Model file for the job. Use its own axes, mm. A direction names the side the tool comes from. Coordinates: 2 decimals unless noted, no trailing zeros. Write each loop counter-clockwise with the first axis right and the second up, starting at its lowest first coordinate (ties: lowest second). Pieces come first, ordered by that corner, then holes. Notation, with made-up numbers: (68, -39) - (109, -39) arc R14 ccw to (109, -12) - close; hole circle Ø11 at (-13.75, -9). An arc over 180 degrees is marked (long way). Put each result on its own line as item: value. Start each with the question number.
1. Which spindle directions (+Z, -Z, +X, -X, +Y, -Y) get a long thin tool onto all of the face, cutting with end or side? Do faces 4 (the face through (-3.53, 4.97, -17.61)), 5 (the face through (2, -2, -13)), 6 (the face through (-2.24, 4.97, -16.63)). Say none if no direction does.
2. Saw through at D-D, the plane x = -1.5. Write the cut outline in (y, z), plus the area to 3 significant figures.
3. Saw through at A-A, the plane x = 0. Write the cut outline in (y, z), plus the area to 3 significant figures.
4. Saw through at B-B, the plane y = 0. Write the cut outline in (x, z).
5. Drill centre lines: L1, parallel to Y at x = 3.5, z = -17; L2, parallel to Z at x = 0, y = -3.9; L3, parallel to Y at x = 2.75, z = -13. Where is each one in solid material? Low to high. Write a range as from..to.
6. Drop flat-ended pins along their axis: P1, Ø1.5, axis at x = -1.5, y = -3, coming from the -Z side; P2, Ø1.5, axis at y = 5, z = -3, coming from the +X side; P3, Ø1.5, axis at x = 1.5, y = -1.5, coming from the -Z side. Give the stop position or say it passes through.
7. Saw through at C-C, the plane z = 4. Write the cut outline in (x, y).
8. Pull direction Y, two halves, no side cores. Call faces 1 (the face through (5.6, 5, -5.1)), 2 (the face through (-0.759, -2.507, -11.583)), 3 (the face through (5.1, -3.2, -16.4)): released by +Y, released by -Y, zero draft, split by the parting line, or undercut.
```python
from build123d import *

# Parameters (mm, degrees)
SKETCH1_W               = 14
SKETCH1_H               = 15
BOSS_EXTRUDE1_DEPTH     = 7
SKETCH3_R               = 4
CUT_EXTRUDE1_DEPTH      = 16
SKETCH4_W               = 14
SKETCH4_H               = 14
BOSS_EXTRUDE2_DEPTH     = 12
SKETCH7_R               = 6
CUT_EXTRUDE7_DEPTH      = 3
SKETCH8_R               = 2.5
CUT_EXTRUDE8_DEPTH      = 11
CUT_EXTRUDE8_DEPTH_BACK = 5
SKETCH9_W               = 4.5
SKETCH9_H               = 6
CUT_EXTRUDE9_DEPTH      = 8
CUT_EXTRUDE9_DEPTH_BACK = 8
CHAMFER1_SIZE           = 5
SKETCH13_R              = 3.5
SKETCH13_R_2            = 2.5
BOSS_EXTRUDE3_DEPTH     = 1
CUT_EXTRUDE10_DEPTH     = 6
CHAMFER2_SIZE           = 4
CHAMFER2_SIZE2          = 2.800830153
CHAMFER2_PART_2_SIZE    = 4
CHAMFER2_PART_2_SIZE2   = 2.800830153
CHAMFER3_SIZE           = 4
CHAMFER3_SIZE2          = 2.800830153
CHAMFER3_PART_2_SIZE    = 4
CHAMFER3_PART_2_SIZE2   = 2.800830153
FILLET1_R               = 1
FILLET2_R               = 4


with BuildPart() as part:
    # Sketch1 → Boss-Extrude1 (new body, symmetric)
    with BuildSketch(Plane(origin=(0, 0, 0), x_dir=(1, 0, 0), z_dir=(0, 1, 0))):
        Rectangle(SKETCH1_W, SKETCH1_H)
    extrude(amount=BOSS_EXTRUDE1_DEPTH, both=True)

    # Sketch3 → Cut-Extrude1 (cut, through all)
    with BuildSketch(Plane.XY.offset(7.5)):
        Circle(SKETCH3_R)
    extrude(amount=-CUT_EXTRUDE1_DEPTH, mode=Mode.SUBTRACT)

    # Sketch4 → Boss-Extrude2 (add)
    with BuildSketch(Plane(origin=(0, 0, -7.5), x_dir=(-1, 0, 0), z_dir=(0, 0, -1))):
        Rectangle(SKETCH4_W, SKETCH4_H)
    extrude(amount=BOSS_EXTRUDE2_DEPTH)

    # Sketch7 → Cut-Extrude7 (cut, symmetric)
    with BuildSketch(Plane(origin=(0, 0, 0), x_dir=(1, 0, 0), z_dir=(0, 1, 0))):
        with Locations((0, 15)):
            Circle(SKETCH7_R)
    extrude(amount=CUT_EXTRUDE7_DEPTH, both=True, mode=Mode.SUBTRACT)

    # Sketch8 → Cut-Extrude8 (cut, two sides)
    with BuildSketch(Plane(origin=(0, -3, 0), x_dir=(1, 0, 0), z_dir=(0, 1, 0))) as cut_extrude8_sk:
        with Locations((0, 15)):
            Circle(SKETCH8_R)
    extrude(amount=CUT_EXTRUDE8_DEPTH, mode=Mode.SUBTRACT)
    extrude(cut_extrude8_sk.sketch, amount=-CUT_EXTRUDE8_DEPTH_BACK, mode=Mode.SUBTRACT)

    # Sketch9 → Cut-Extrude9 (cut, two sides)
    with BuildSketch(Plane(origin=(0, 0, 0), x_dir=(0, 0, -1), z_dir=(1, 0, 0))) as cut_extrude9_sk:
        with Locations((17.25, 0)):
            Rectangle(SKETCH9_W, SKETCH9_H)
    extrude(amount=CUT_EXTRUDE9_DEPTH, mode=Mode.SUBTRACT)
    extrude(cut_extrude9_sk.sketch, amount=-CUT_EXTRUDE9_DEPTH_BACK, mode=Mode.SUBTRACT)

    # Chamfer1
    chamfer1_edges = [part.edges().sort_by_distance(p)[0] for p in [
        (7, -5, -19.5),
        (-7, -5, -19.5),
    ]]
    chamfer(chamfer1_edges, length=CHAMFER1_SIZE)

    # Sketch13 → Boss-Extrude3 (add)
    with BuildSketch(Plane(origin=(0, -3, 0), x_dir=(1, 0, 0), z_dir=(0, 1, 0))):
        with Locations((0, 15)):
            Circle(SKETCH13_R)
        with Locations((0, 15)):
            Circle(SKETCH13_R_2, mode=Mode.SUBTRACT)
    extrude(amount=BOSS_EXTRUDE3_DEPTH)

    # Sketch14 → Cut-Extrude10 (cut)
    with BuildSketch(Plane(origin=(0, 7, 0), x_dir=(1, 0, 0), z_dir=(0, 1, 0))):
        Polygon((0, 15), (11.277541362, 24.462980798), (-11.751290712, 24.860503702), align=None)
    extrude(amount=-CUT_EXTRUDE10_DEPTH, mode=Mode.SUBTRACT)

    # Chamfer2
    chamfer2_edges = [part.edges().sort_by_distance(p)[0] for p in [
        (7, 7, -3.5),
    ]]
    chamfer2_side = [part.faces().sort_by_distance(p)[0] for p in [
        (7, 0, -3.5),
    ]]
    chamfer(chamfer2_edges, length=CHAMFER2_SIZE, length2=CHAMFER2_SIZE2, reference=chamfer2_side[0])

    # Chamfer2 part 2
    chamfer2_part_2_edges = [part.edges().sort_by_distance(p)[0] for p in [
        (-7, 7, -3.5),
    ]]
    chamfer2_part_2_side = [part.faces().sort_by_distance(p)[0] for p in [
        (-7, 0, -3.5),
    ]]
    chamfer(chamfer2_part_2_edges, length=CHAMFER2_PART_2_SIZE, length2=CHAMFER2_PART_2_SIZE2, reference=chamfer2_part_2_side[0])

    # Chamfer3
    chamfer3_edges = [part.edges().sort_by_distance(p)[0] for p in [
        (7, -7, -3.5),
    ]]
    chamfer3_side = [part.faces().sort_by_distance(p)[0] for p in [
        (7, -2, -3.5),
    ]]
    chamfer(chamfer3_edges, length=CHAMFER3_SIZE, length2=CHAMFER3_SIZE2, reference=chamfer3_side[0])

    # Chamfer3 part 2
    chamfer3_part_2_edges = [part.edges().sort_by_distance(p)[0] for p in [
        (-7, -7, -3.5),
    ]]
    chamfer3_part_2_side = [part.faces().sort_by_distance(p)[0] for p in [
        (-7, -2, -3.5),
    ]]
    chamfer(chamfer3_part_2_edges, length=CHAMFER3_PART_2_SIZE, length2=CHAMFER3_PART_2_SIZE2, reference=chamfer3_part_2_side[0])

    # Fillet1
    fillet1_edges = [part.edges().sort_by_distance(p)[0] for p in [
        (-3.534338156, 5, -17.965661844),
        (3.534338156, 5, -17.965661844),
        (1.915111108, 5, -16.606969024),
        (-1.915111108, 5, -16.606969024),
    ]]
    fillet(fillet1_edges, radius=FILLET1_R)

    # Fillet2
    fillet2_edges = [part.edges().sort_by_distance(p)[0] for p in [
        (-2, -5, -19.5),
        (2, -5, -19.5),
    ]]
    fillet(fillet2_edges, radius=FILLET2_R)


solid = part.part
```
Final values:
1. face 4: -Z, +Y
1. face 5: -Z
1. face 6: +Y
2. outline: (-7, -19.33) - (-3, -19.33) - (-3, -18.16) - (-2, -18.16) - (-2, -17) - (-7, -17) - close; (-7, -13) - (-2, -13) - (-2, -11.84) - (-3, -11.84) - (-3, -9.19) - (3, -9.19) - (3, -13) - (7, -13) - (7, 7.5) - (3.71, 7.5) - (3.71, -7.5) - (-3.71, -7.5) - (-3.71, 7.5) - (-7, 7.5) - close
2. area: 165 mm²
3. outline: (-7, -19.5) - (-3, -19.5) - (-3, -18.5) - (-2, -18.5) - (-2, -17.5) - (-7, -17.5) - close; (-7, -12.5) - (-2, -12.5) - (-2, -11.5) - (-3, -11.5) - (-3, -9) - (3, -9) - (3, -12.5) - (7, -12.5) - (7, 7.5) - (4, 7.5) - (4, -7.5) - (-4, -7.5) - (-4, 7.5) - (-7, 7.5) - close
3. area: 149 mm²
4. outline: (-7, -14.5) - (-6.5, -15) - (-6, -15) arc R6 cw to (6, -15) - (6.5, -15) - (7, -14.5) - (7, 7.5) - (4, 7.5) - (4, -7.5) - (-4, -7.5) - (-4, 7.5) - (-7, 7.5) - close
5. L1: y = -7..-3, 3..7
5. L2: z = -19.5..-17.5, -12.5..-7.5
5. L3: y = -7..-2, 3..7
6. P1: stops at z = -19.48
6. P2: stops at x = 6.12
6. P3: stops at z = -18.37
7. outline: (-7, -3) - (-4.2, -7) - (4.2, -7) - (7, -3) - (7, 3) - (4.2, 7) - (-4.2, 7) - (-7, 3) - close; hole circle Ø8 at (0, 0)
8. face 1: released by +Y
8. face 2: undercut
8. face 3: zero draft
